Could you check a few things on this model? Use its own coordinates, in mm. Coordinates: 2 decimals unless noted, no trailing zeros. Loops run counter-clockwise (first coordinate to the right, second up) from the corner with the lowest first, then second, coordinate; pieces in that order, holes last.
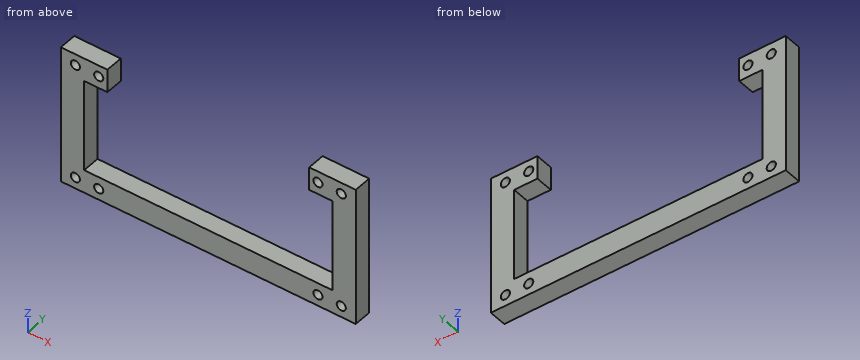
from build123d import *

# Parameters (mm, degrees)
SKETCH1_R           = 1.651
BOSS_EXTRUDE1_DEPTH = 6.35


with BuildPart() as part:
    # Sketch1 → Boss-Extrude1 (new body)
    with BuildSketch(Plane(origin=(0, 0, 0), x_dir=(1, 0, 0), z_dir=(0, 1, 0))):
        Polygon((75.155177047, 61.997896552), (75.155177047, 11.997896552), (91.919177047, 11.997896552), (91.919177047, 20.379896552), (83.537177047, 20.379896552), (83.537177047, 53.615896552), (173.037829354, 53.615896552), (173.037829354, 20.379896552), (164.655829354, 20.379896552), (164.655829354, 11.997896552), (181.419829354, 11.997896552), (181.419829354, 61.997896552), align=None)
        with Locations((80.3721812, 16.064784874)):
            Circle(SKETCH1_R, mode=Mode.SUBTRACT)
        with Locations((80.3721812, 57.93100823)):
            Circle(SKETCH1_R, mode=Mode.SUBTRACT)
        with Locations((88.7874552, 16.064784874)):
            Circle(SKETCH1_R, mode=Mode.SUBTRACT)
        with Locations((167.7875512, 57.93100823)):
            Circle(SKETCH1_R, mode=Mode.SUBTRACT)
        with Locations((88.7874552, 57.93100823)):
            Circle(SKETCH1_R, mode=Mode.SUBTRACT)
        with Locations((176.2028252, 57.93100823)):
            Circle(SKETCH1_R, mode=Mode.SUBTRACT)
        with Locations((176.2028252, 16.064784874)):
            Circle(SKETCH1_R, mode=Mode.SUBTRACT)
        with Locations((167.7875512, 16.064784874)):
            Circle(SKETCH1_R, mode=Mode.SUBTRACT)
    extrude(amount=BOSS_EXTRUDE1_DEPTH)


solid = part.part
1) If I drill on L1, parallel to X at y = 5, z = -47.5; L2, parallel to X at y = 1.75, z = -58.5; L3, parallel to Z at x = 88, y = 4.25, over which ranges is the centre line in solid material (lowest first)?
2) Imagine slicing it at A-A on x = 171. List the corners of the cut face in (y, z) for me.
3) Imagine slicing it at D-D on x = 120.5. List the corners of the cut face in (y, z) for me.
4) Imagine slicing it at B-B on z = -43. List the corners of the cut face in (x, y) for me.
5) Will this pin go through, and if not, where does the flat tip stop? pin 1 (2 mm diameter, centred on x = 119.5, y = 3.5, fed in from +Z).
6) Imagine slicing it at C-C on y = 2.5. State how many separate pieces and enclosed holes the cut face has, plus the area to 3 significant figures.
Solved:
1. L1: x = 75.16 to 83.54, 173.04 to 181.42
1. L2: x = 75.16 to 78.82, 81.92 to 87.24, 90.34 to 166.24, 169.34 to 174.65, 177.75 to 181.42
1. L3: z = -62 to -59.38, -56.48 to -53.62, -20.38 to -17.52, -14.61 to -12
2. outline: (0, -62) - (6.35, -62) - (6.35, -53.62) - (0, -53.62) - close; (0, -20.38) - (6.35, -20.38) - (6.35, -12) - (0, -12) - close
3. outline: (0, -62) - (6.35, -62) - (6.35, -53.62) - (0, -53.62) - close
4. outline: (75.16, 0) - (83.54, 0) - (83.54, 6.35) - (75.16, 6.35) - close; (173.04, 0) - (181.42, 0) - (181.42, 6.35) - (173.04, 6.35) - close
5. pin 1: stops at z = -53.62
6. separate pieces: 1
6. enclosed holes: 8
6. area: 1,660 mm2
